Autodesk Inventor part; units mm, degrees
ref_plane "YZ Plane" through (0, 0, 0) normal (1, 0, 0) x (0, 1, 0)
ref_plane "XZ Plane" through (0, 0, 0) normal (0, 1, 0) x (-1, 0, 0)
ref_plane "XY Plane" through (0, 0, 0) normal (0, 0, 1) x (1, 0, 0)
sketch "Эскиз1" plane through (0, 0, 0) normal (0, 0, 1) x (1, 0, 0)
  line L0 (0, 0) -> (6, 0)
  line L1 (6, 0) -> (6, 38)
  line L2 (6, 38) -> (0, 38)
  line L3 (0, 38) -> (0, 0)
  line L4 (0, 0) -> (49.5, 0)
  line L5 (49.5, 0) -> (49.5, 5)
  line L6 (49.5, 5) -> (0, 5)
  line L7 (0, 5) -> (0, 0)
  line L8 (49.5, 0) -> (55.5, 0) construction
  line L9 (55.5, 0) -> (55.5, 38) construction
  line L10 (55.5, 38) -> (49.5, 38)
  line L11 (49.5, 38) -> (49.5, 0)
  line L12 (49.5, 0) -> (71, 24.2678)
  line L13 (71, 24.2678) -> (55.5, 38)
  dimension "d0" = 5
  dimension "d1" = 6
  dimension "d2" = 43.5
  dimension "d3" = 6
  dimension "d4" = 38
  dimension "d5" = 38
  dimension "d6" = 71
  dimension "d7" = 90
extrude "Выдавливание1" add sketch "Эскиз1" along normal blind 20.5
sketch "Эскиз2" plane through (0, 0, 0) normal (0, 0, -1) x (-1, 0, 0)
  line L0 (-49.5, 0) -> (-71, 24.2678)
  line L1 (-71, 24.2678) -> (-57.4058, 8.9235)
  line L2 (-57.4058, 8.9235) -> (-52.9148, 12.9023)
  line L3 (-52.9148, 12.9023) -> (-66.509, 28.2466)
  line L4 (-66.509, 28.2466) -> (-71, 24.2678)
  line L5 (-71, 24.2678) -> (-55.5, 38)
  line L6 (-58.6417, 14.8426) -> (-55.1603, 10.9129)
  line L7 (-65.273, 22.3276) -> (-68.7545, 26.2572)
  circle A0 centre (-65.273, 22.3276) radius 1
  circle A1 centre (-58.6417, 14.8426) radius 1
  point P0 (0, 0)
  dimension "d10" = 6
  dimension "d11" = 20.5
  dimension "d13" = 2
  dimension "d14" = 2
  dimension "d15" = 8
extrude "Выдавливание2" add sketch "Эскиз2" along normal blind 7
sketch "Эскиз3" plane through (49.5, 38, 0) normal (0, 1, 0) x (1, 0, 0)
  circle A0 centre (3, -5.25) radius 1
  circle A1 centre (3, -15.25) radius 1
  circle A2 centre (-46.5, -5.25) radius 1
  circle A3 centre (-46.5, -15.25) radius 1
  line L0 (6, -20.5) -> (0, -20.5)
  line L1 (3, -5.25) -> (3, -15.25) construction
  line L2 (6, 0) -> (6, -20.5)
  line L3 (-43.5, 0) -> (-49.5, 0)
  line L4 (0, 0) -> (0, -20.5)
  circle A4 centre (-12, -10.25) radius 2
  point P0 (3, -20.5)
  point P1 (3, -10.25)
  point P2 (6, -10.25)
  point P3 (-46.5, 0)
  point P4 (6, -10.25)
  dimension "d18" = 2
  dimension "d19" = 10
  dimension "d20" = 4
  dimension "d21" = 18
extrude "Выдавливание3" cut sketch "Эскиз3" against normal up to next contours A4
extrude "Выдавливание4" cut sketch "Эскиз3" against normal blind 15 contours A0 | A1 | A2 | A3
sketch "Эскиз4" plane through (55.5, 38, 20.5) normal (0.6631, 0.7485, 0) x (0.7485, -0.6631, 0)
  circle A0 centre (7.958, 10.25) radius 5.75
  line L0 (0, 20.5) -> (0, 0)
  line L1 (20.708, 27.5) -> (20.708, 0)
  point P0 (-16.3428, 20.5)
  point P1 (0, 10.25)
  dimension "d26" = 7
  dimension "d27" = 11.5
extrude "Выдавливание5" cut sketch "Эскиз4" against normal up to next
sketch "Эскиз5" plane through (0, 0, 0) normal (0, -1, 0) x (1, 0, 0)
  circle A0 centre (48.25, 10.25) radius 5.75
  line L0 (49.5, 0) -> (49.5, 20.5)
  circle A1 centre (37.5, 10.25) radius 2
  point P0 (0, 0)
  point P1 (49.5, 10.25)
  dimension "d30" = 11.5
  dimension "d31" = 3
extrude "Выдавливание6" cut sketch "Эскиз5" against normal up to next contours A0 L0 | L0 A0
properties part number "kreplenie3"
Can you work these out from the model? Positions are in its coordinate system, mm. A direction names the side the tool comes from. Coordinates: 2 decimals unless noted, no trailing zeros. Write each loop counter-clockwise with the first axis right and the second up, starting at its lowest first coordinate (ties: lowest second). Pieces come first, ordered by that corner, then holes. Notation, with made-up numbers: M -39,28.5 L 18,28.5 A16 ccw 18,33.5 Z; hole C 64.5,-2.75 d7. An arc over 180 degrees is marked long. Answer as CSV lines item,"result".
Item 1: I'm going to push flat-ended pins straight in: P1, Ø1.6, axis at x = 3, z = 5.25, coming from the +Y side; P2, Ø3, axis at x = 62.5, y = 30, coming from the -Z side; P3, Ø8, axis at x = 39.5, y = 11.5, coming from the +Z side; P4, Ø1.5, axis at x = 56.5, z = 17, coming from the -Y side. Where does each tip first touch, or does it pass through?
Geometry results:
P1,"stops at y = 23"
P2,"stops at z = 0"
P3,"passes through"
P4,"stops at y = 7.05"
Item 2: Imagine slicing it at C-C on x = 3. List the corners of the cut face in (y, z) for me, plus the area to 3 significant figures.
Geometry results:
outline,"M 0,0 L 38,0 L 38,4.25 L 23,4.25 L 23,6.25 L 38,6.25 L 38,14.25 L 23,14.25 L 23,16.25 L 38,16.25 L 38,20.5 L 0,20.5 Z"
area,"719 mm2"
Item 3: Imagine slicing it at D-D on z = 1.75. List the corners of the cut face in (x, y) for me.
Geometry results:
outline,"M 0,0 L 49.5,0 L 71,24.27 L 55.5,38 L 49.5,38 L 49.5,5 L 6,5 L 6,38 L 0,38 Z"
Item 4: We'd pull the mould along Y, two halves only. Please class faces 1 (the flat face through (0, 19, 10)), 2 (the flat face through (59.62, 20.47, -3.45)), 3 (the cylindrical face through (60.64, 23.53, 8.52)), 4 (the cylindrical face through (64.32, 22.03, -3.45)): +Y half, -Y half, draft (parallel to the pull), parting line (faces both ways), or undercut.
Geometry results:
face 1,"draft"
face 2,"+Y half"
face 3,"undercut"
face 4,"undercut"
Item 5: On a 3-axis mill with a long thin cutter (end or side, diameter ignored), from which of +Z, -Z, +X, -X, +Y, -Y can I reach the whole of each face in a straight line? I mean faces 5 (the flat face through (59, 15, 0)), 6 (the flat face through (55.192, 10.885, -3.451)), 7 (the cylindrical face through (2.87, 30.6, 4.26)). Say none if no direction works.
Geometry results:
face 5,"-Z"
face 6,"-Z, -X, -Y"
face 7,"+Y"
Item 6: Imagine slicing it at B-B on z = 10.25. List the corners of the cut face in (x, y) for me, plus the area to 3 significant figures.
Geometry results:
outline,"M 0,0 L 35.5,0 L 35.5,5 L 6,5 L 6,38 L 0,38 Z; M 39.5,0 L 42.5,0 L 42.5,5 L 39.5,5 Z; M 49.5,27.9 L 57.15,36.54 L 55.5,38 L 49.5,38 Z; M 54,5.08 L 71,24.27 L 65.76,28.91 L 54,15.63 Z"
area,"585 mm2"
Item 7: Imagine slicing it at A-A on x = 48.25. List the corners of the cut face in (y, z) for me, plus the area to 3 significant figures.
Geometry results:
outline,"M 0,0 L 5,0 L 5,4.5 L 0,4.5 Z; M 0,16 L 5,16 L 5,20.5 L 0,20.5 Z"
area,"45.0 mm2"
Item 8: Please list where these lines run through material, in increasing order: line 1 along X through (y, z) = (32, 14.75); line 2 along X through (y, z) = (29.75, 15.25); line 3 along X through (y, z) = (34, 15.25).
Geometry results:
line 1,"x = 0 to 2.13, 3.87 to 6, 49.5 to 51.63, 53.37 to 56.03"
line 2,"x = 0 to 2, 4 to 6, 49.5 to 51.5, 53.5 to 55.03, 62.62 to 64.81"
line 3,"x = 0 to 2, 4 to 6, 49.5 to 51.5, 53.5 to 58.79"
